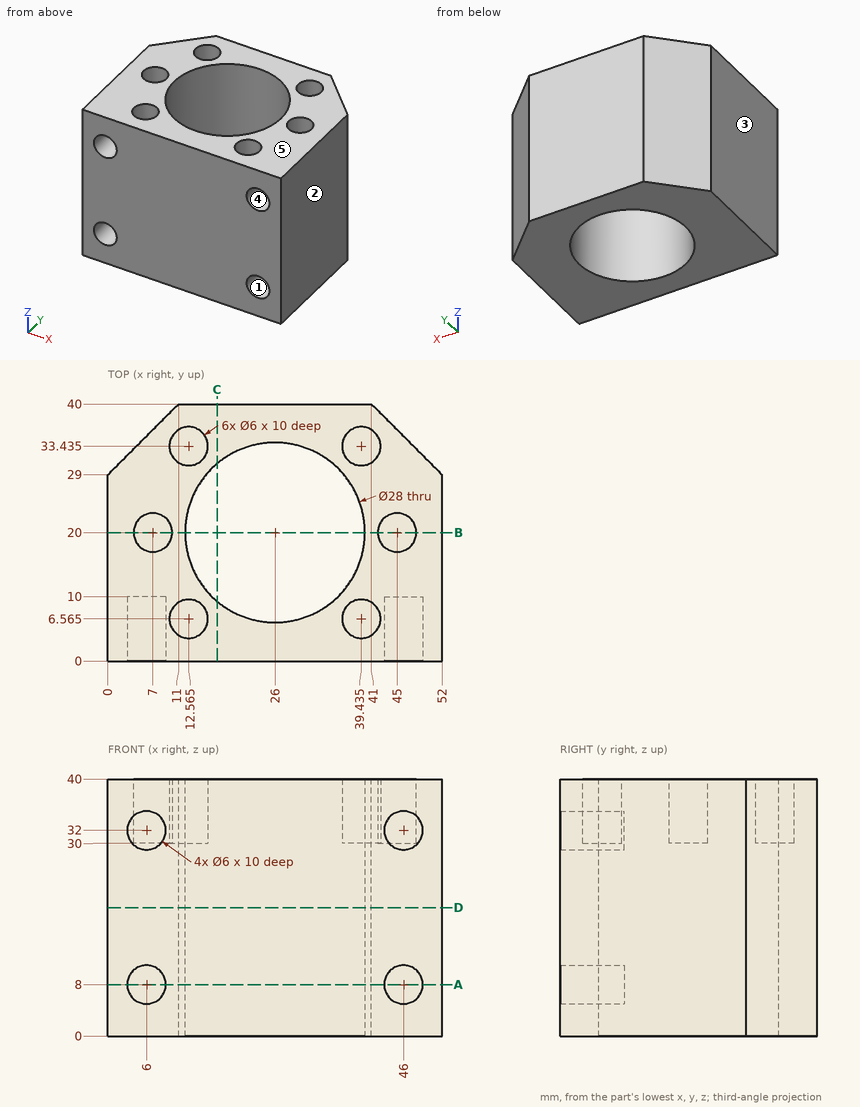
Can you work these out from the drawing? Everything is in mm from the part's minimum corner. A direction names the side the tool comes from. Round coordinates to 2 decimals unless told otherwise and drop trailing zeros. Loops run counter-clockwise (first coordinate to the right, second up) from the corner with the lowest first, then second, coordinate; pieces in that order, holes last. Notation, with made-up numbers: (-38, 78) - (2, 78) arc R12 cw to (2, 98) - close; hole circle Ø9 at (-2.5, -4). An arc over 180 degrees is marked (long way). Answer in a Markdown table with one row per item. Add a question column.
(1) I need wall thicknesses on line 1 along X through (y, z) = (19, 35.5); line 2 along Y through (x, z) = (26, 8); line 3 along Z through (x, y) = (40.5, 8). Which ranges of each line are inside material? Lowest first, please.
(2) If we mould it in two halves opening along Z, with no side actions, what happens to the marked faces 3, 4 and 5? For each: pulls with the +Z half, pulls with the -Z half, needs draft (parallel to the pull), parting line crosses it, or undercut.
(3) If we section it at D-D (z = 20): Please give me the cut outline in (x, y), plus the area to 3 significant figures.
(4) I'm going to push flat-ended pins straight in: pin 1 (3 mm diameter, centred on x = 5.5, z = 7.5, fed in from -Y); pin 2 (1.5 mm diameter, centred on x = 7, z = 17, fed in from +Y); pin 3 (3 mm diameter, centred on x = 12, y = 7, fed in from +Z); pin 4 (1.5 mm diameter, centred on x = 32.5, y = 31, fed in from -Z). Where does each tip first touch, or does it pass through?
(5) For the marked faces 1 and 2, which set-ups out of +Z, -Z, +X, -X, +Y, -Y let a thin tool reach every point of the face, with its end or its side?
(6) If we section it at B-B (y = 20): Please give me the cut outline in (x, z), plus the area to 3 significant figures.
(7) If we section it at C-C (x = 17): Please give me the cut outline in (y, z).
(8) If we section it at A-A (z = 8): Please give me the cut outline in (x, y), plus the area to 3 significant figures.
Model answer:
| question | item | result |
|---|---|---|
| 1 | line 1 | x = 0 to 4.17, 9.83 to 12.04, 39.96 to 42.17, 47.83 to 52 |
| 1 | line 2 | y = 0 to 6, 34 to 40 |
| 1 | line 3 | z = 0 to 30 |
| 2 | face 3 | needs draft |
| 2 | face 4 | undercut |
| 2 | face 5 | pulls with the +Z half |
| 3 | outline | (0, 0) - (52, 0) - (52, 29) - (41, 40) - (11, 40) - (0, 29) - close; hole circle Ø28 at (26, 20) |
| 3 | area | 1,340 mm² |
| 4 | pin 1 | stops at y = 10 |
| 4 | pin 2 | stops at y = 36.75 |
| 4 | pin 3 | stops at z = 30 |
| 4 | pin 4 | passes through |
| 5 | face 1 | -Y |
| 5 | face 2 | +Z, -Z, +X, +Y, -Y |
| 6 | outline | (0, 0) - (12, 0) - (12, 40) - (10, 40) - (10, 30) - (4, 30) - (4, 40) - (0, 40) - close; (40, 0) - (52, 0) - (52, 40) - (48, 40) - (48, 30) - (42, 30) - (42, 40) - (40, 40) - close |
| 6 | area | 840 mm² |
| 7 | outline | (0, 0) - (9.28, 0) - (9.28, 40) - (0, 40) - close; (30.72, 0) - (40, 0) - (40, 40) - (30.72, 40) - close |
| 8 | outline | (0, 0) - (3, 0) - (3, 10) - (9, 10) - (9, 0) - (43, 0) - (43, 10) - (49, 10) - (49, 0) - (52, 0) - (52, 29) - (41, 40) - (11, 40) - (0, 29) - close; hole circle Ø28 at (26, 20) |
| 8 | area | 1,220 mm² |
